The model under review builds one solid part; all positions refer to its coordinate system, in mm. Face numbers are marked on the shaded views. A direction names the side the tool comes from. Give positions to 0.01 mm unless a question says otherwise; leave off trailing zeros. Order: outer loops, then holes, each group sorted by start corner. A loop starts at its lowest first (then second) coordinate and runs counter-clockwise, first axis right, second up.
```python
from build123d import *

# Parameters (mm, degrees)
F1_DEPTH = 4.318
F2_R     = 13.8522977146
F3_DEPTH = 6.096


with BuildPart() as f1:
    # F0 (on Front) → F1 (new body)
    with BuildSketch(Plane.XZ):
        with BuildLine():
            Line((6.0770163177, 33.1509892084), (-25.6710906561, 21.8383451146))
            Line((-25.6710906561, 21.8383451146), (-12.8355453281, 10.9191725573))
            ThreePointArc((-12.8355453281, 10.9191725573), (-5.6563220469, 15.8740534869), (3.0385081589, 16.5754946042))
            Line((3.0385081589, 16.5754946042), (6.0770163177, 33.1509892084))
        make_face()
        Polygon((-15.8740534869, -5.6563220469), (-25.6710906561, 21.8383451146), (-31.7481069739, -11.3126440938), align=None)
        with BuildLine():
            Line((31.7481069739, 11.3126440938), (6.0770163177, 33.1509892084))
            Line((6.0770163177, 33.1509892084), (3.0385081589, 16.5754946042))
            ThreePointArc((3.0385081589, 16.5754946042), (10.9191725573, 12.8355453281), (15.8740534869, 5.6563220469))
            Line((15.8740534869, 5.6563220469), (31.7481069739, 11.3126440938))
        make_face()
        with BuildLine():
            Line((25.6710906561, -21.8383451146), (31.7481069739, 11.3126440938))
            Line((31.7481069739, 11.3126440938), (15.8740534869, 5.6563220469))
            ThreePointArc((15.8740534869, 5.6563220469), (16.6054844473, 2.8700939835), (16.8516928884, 0))
            ThreePointArc((16.8516928884, 0), (10.7883165247, -12.9457243818), (-3.0385081589, -16.5754946042))
            Line((-3.0385081589, -16.5754946042), (-6.0770163177, -33.1509892084))
            Line((-6.0770163177, -33.1509892084), (25.6710906561, -21.8383451146))
        make_face()
        with BuildLine():
            Line((-15.8740534869, -5.6563220469), (-31.7481069739, -11.3126440938))
            Line((-31.7481069739, -11.3126440938), (-6.0770163177, -33.1509892084))
            Line((-6.0770163177, -33.1509892084), (-3.0385081589, -16.5754946042))
            ThreePointArc((-3.0385081589, -16.5754946042), (-10.9191725573, -12.8355453281), (-15.8740534869, -5.6563220469))
        make_face()
        with BuildLine():
            ThreePointArc((15.8740534869, 5.6563220469), (10.9191725573, 12.8355453281), (3.0385081589, 16.5754946042))
            Line((3.0385081589, 16.5754946042), (0, 0))
            Line((0, 0), (15.8740534869, 5.6563220469))
        make_face()
        with BuildLine():
            ThreePointArc((3.0385081589, 16.5754946042), (-5.6563220469, 15.8740534869), (-12.8355453281, 10.9191725573))
            Line((-12.8355453281, 10.9191725573), (0, 0))
            Line((0, 0), (3.0385081589, 16.5754946042))
        make_face()
        with BuildLine():
            Line((0, 0), (-12.8355453281, 10.9191725573))
            ThreePointArc((-12.8355453281, 10.9191725573), (-16.5754946042, 3.0385081589), (-15.8740534869, -5.6563220469))
            Line((-15.8740534869, -5.6563220469), (0, 0))
        make_face()
        with BuildLine():
            Line((-12.8355453281, 10.9191725573), (-25.6710906561, 21.8383451146))
            Line((-25.6710906561, 21.8383451146), (-15.8740534869, -5.6563220469))
            ThreePointArc((-15.8740534869, -5.6563220469), (-16.5754946042, 3.0385081589), (-12.8355453281, 10.9191725573))
        make_face()
        with BuildLine():
            Line((0, 0), (-15.8740534869, -5.6563220469))
            ThreePointArc((-15.8740534869, -5.6563220469), (-10.9191725573, -12.8355453281), (-3.0385081589, -16.5754946042))
            Line((-3.0385081589, -16.5754946042), (0, 0))
        make_face()
        with BuildLine():
            Line((15.8740534869, 5.6563220469), (0, 0))
            Line((0, 0), (-3.0385081589, -16.5754946042))
            ThreePointArc((-3.0385081589, -16.5754946042), (10.7883165247, -12.9457243818), (16.8516928884, 0))
            ThreePointArc((16.8516928884, 0), (16.6054844473, 2.8700939835), (15.8740534869, 5.6563220469))
        make_face()
    extrude(amount=F1_DEPTH)

    # F2 (on face) → F3 (join)
    with BuildSketch(Plane.XZ.offset(4.318)):
        with Locations((2.9549675528, 2.9199353885)):
            Circle(F2_R)
    extrude(amount=F3_DEPTH)


solid = f1.part
```
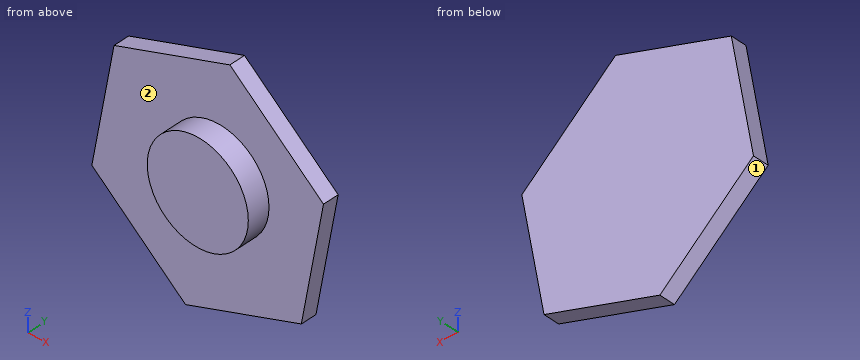
Item 1: For line 1 (Y direction, x = 17, z = 8); line 2 (X direction, y = -7.5, z = 3.5); line 3 (Z direction, x = -14, y = -1.75), list the stretches that pass through material, from the lowest coordinate up.
Values found:
line 1: y = -4.32 to 0
line 2: x = -10.89 to 16.8
line 3: z = -26.41 to 26
Item 2: For the marked faces 1 and 2, list the 3-axis set-ups (+Z, -Z, +X, -X, +Y, -Y) from which the entire face can be reached by the end or side of a thin tool; tool diameter is ignored.
Values found:
face 1: -Z, -X, +Y, -Y
face 2: -Y
Item 3: Take a section at B-B (y = -2.5). Give the boundary of the cut face in (x, z), and give its area (3 significant figures).
Values found:
outline: (-31.75, -11.31) - (-6.08, -33.15) - (25.67, -21.84) - (31.75, 11.31) - (6.08, 33.15) - (-25.67, 21.84) - close
area: 2,950 mm2
Item 4: Take a section at C-C (z = 4.5). Give the boundary of the cut face in (x, y), and give its area (3 significant figures).
Values found:
outline: (-28.85, -4.32) - (-10.81, -4.32) - (-10.81, -10.41) - (16.72, -10.41) - (16.72, -4.32) - (30.5, -4.32) - (30.5, 0) - (-28.85, 0) - close
area: 424 mm2
Item 5: Take a section at D-D (x = 21). Give the boundary of the cut face in (y, z).
Values found:
outline: (-4.32, -23.5) - (0, -23.5) - (0, 20.46) - (-4.32, 20.46) - close
Item 6: Take a section at A-A (x = -4.5). Give the boundary of the cut face in (y, z).
Values found:
outline: (-10.41, -8.76) - (-4.32, -8.76) - (-4.32, -32.59) - (0, -32.59) - (0, 29.38) - (-4.32, 29.38) - (-4.32, 14.6) - (-10.41, 14.6) - close
Item 7: Clearance check with flat-ended pins moving along their axes: pin 1 Ø4 at (x, z) = (10, 1.5) entering from +Y; pin 2 Ø1.5 at (x, y) = (-11, -3.5) entering from +Z; pin 3 Ø4 at (x, y) = (15.5, -3) entering from +Z; pin 4 Ø4 at (x, y) = (-6.5, -7) entering from -Z. State where each tip first meets the part, or that it passes through.
Values found:
pin 1: stops at y = 0
pin 2: stops at z = 27.33
pin 3: stops at z = 26.84
pin 4: stops at z = -8.76
